from build123d import *

# Parameters (mm, degrees)
SKETCH1_W                       = 16
SKETCH1_H                       = 8
BOSS_EXTRUDE1_DEPTH             = 3
SHELL3_T                        = -1
SKETCH2_R                       = 1.5
SKETCH2_R_2                     = 0.8
BOSS_EXTRUDE2_DEPTH             = 2
BOSS_EXTRUDE3_DEPTH             = 11
CUT_EXTRUDE2_DEPTH              = 10
SKETCH5_R                       = 1.2
BOSS_EXTRUDE4_DEPTH             = 5
BOSS_EXTRUDE4_DIRECTION_2_REACH = 32.577


with BuildPart() as part:
    # Sketch1 → Boss-Extrude1 (new body)
    with BuildSketch(Plane.XY):
        with Locations((-13.569515058, 18.04477027)):
            Rectangle(SKETCH1_W, SKETCH1_H)
    extrude(amount=BOSS_EXTRUDE1_DEPTH)

    # Shell3
    shell3_openings = [part.faces().sort_by_distance(p)[0] for p in [
        (-13.569515058, 18.04477027, 0),
    ]]
    offset(amount=SHELL3_T, openings=shell3_openings, kind=Kind.INTERSECTION)

    # Sketch2 → Boss-Extrude2 (add)
    with BuildSketch(Plane(origin=(0, 0, 2), x_dir=(-1, 0, 0), z_dir=(0, 0, -1))):
        with Locations((13.569515058, 18.04477027)):
            Circle(SKETCH2_R)
        with Locations((13.569515058, 18.04477027)):
            Circle(SKETCH2_R_2, mode=Mode.SUBTRACT)
    extrude(amount=BOSS_EXTRUDE2_DEPTH)

    # Sketch3 → Boss-Extrude3 (add)
    with BuildSketch(Plane.XY.offset(3)):
        with BuildLine():
            Line((-17.569515058, 22.04477027), (-17.569515058, 20.54477027))
            Line((-17.569515058, 20.54477027), (-15.569515058, 20.54477027))
            ThreePointArc((-15.569515058, 20.54477027), (-13.569515058, 19.54477027), (-11.569515058, 20.54477027))
            Line((-11.569515058, 20.54477027), (-9.569515058, 20.54477027))
            Line((-9.569515058, 20.54477027), (-9.569515058, 22.04477027))
            Line((-9.569515058, 22.04477027), (-17.569515058, 22.04477027))
        make_face()
    extrude(amount=BOSS_EXTRUDE3_DEPTH)

    # Sketch4 → Cut-Extrude2 (cut)
    with BuildSketch(Plane.ZY.offset(17.569515058)):
        Polygon((14, 21.29477027), (14, 19.54477027), (10, 19.54477027), align=None)
    extrude(amount=-CUT_EXTRUDE2_DEPTH, mode=Mode.SUBTRACT)

    # Sketch5 → Boss-Extrude4 (add)
    with BuildSketch(Plane(origin=(0, 12.732659637, -5.570538591), x_dir=(-1, 0, 0), z_dir=(0, -0.9161573349021893, 0.4008188340197074))):
        with Locations(Location((13.569515058, -20.425962901, 0), (0, 0, 90))):
            Circle(SKETCH5_R)
    extrude(amount=BOSS_EXTRUDE4_DEPTH)

    # Sketch5 → Boss-Extrude4 direction 2 (add, up to next)
    with BuildSketch(Plane(origin=(0, 12.732659637, -5.570538591), x_dir=(-1, 0, 0), z_dir=(0, -0.9161573349021893, 0.4008188340197074)), mode=Mode.PRIVATE) as boss_extrude4_direction_2_sk1:
        with Locations(Location((13.569515058, -20.425962901, 0), (0, 0, 90))):
            Circle(SKETCH5_R)
    boss_extrude4_direction_2_tool1 = extrude(boss_extrude4_direction_2_sk1.sketch, amount=-BOSS_EXTRUDE4_DIRECTION_2_REACH, mode=Mode.PRIVATE) - part.part
    add(boss_extrude4_direction_2_tool1.solids().sort_by_distance((-13.569515, 20.91977, 13.142857))[0])


solid = part.part
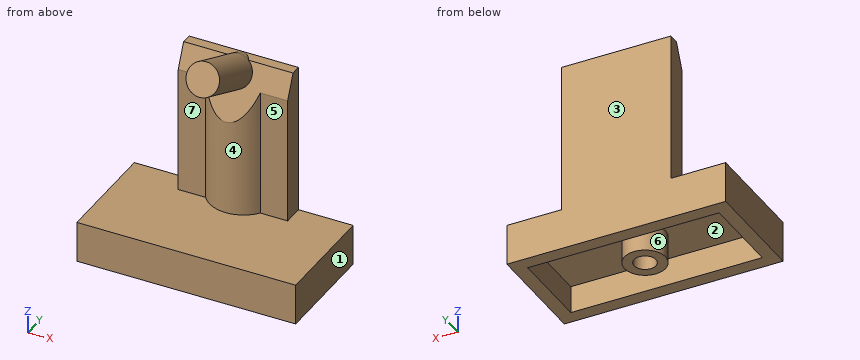
Read the model definition and answer for the solid it produces. Units are mm, in the model's axes. Face numbers are marked on the shaded views. A direction names the side the tool comes from. Coordinates: 2 decimals unless noted, no trailing zeros. Loops run counter-clockwise (first coordinate to the right, second up) from the corner with the lowest first, then second, coordinate; pieces in that order, holes last. Notation, with made-up numbers: (49.25, -32) - (98.25, -32) arc R30 ccw to (98.25, -8) - close; hole circle Ø10 at (-30, 87.5). An arc over 180 degrees is marked (long way). Answer in a Markdown table with one row per item.
Q1. Find section B-B on z = 6.25. Write down the section's boundary in (x, y).
Here are the results:
| item | result |
|---|---|
| outline | (-17.57, 20.54) - (-15.57, 20.54) arc R2.5 ccw to (-11.57, 20.54) - (-9.57, 20.54) - (-9.57, 22.04) - (-17.57, 22.04) - close |
Q2. Find section C-C on x = -19.5. Write down the section's boundary in (y, z), plus the area to 3 significant figures.
Here are the results:
| item | result |
|---|---|
| outline | (14.04, 0) - (15.04, 0) - (15.04, 2) - (21.04, 2) - (21.04, 0) - (22.04, 0) - (22.04, 3) - (14.04, 3) - close |
| area | 12.0 mm^2 |
Q3. The mould has two halves that part along Y. Classify the marked faces 1, 2 and 3: pulls with the +Y half, pulls with the -Y half, needs draft (parallel to the pull), parting line crosses it, or undercut.
Here are the results:
| item | result |
|---|---|
| face 1 | needs draft |
| face 2 | undercut |
| face 3 | pulls with the +Y half |
Q4. For the marked faces 4, 5, 6 and 7, determine the directions among +Z, -Z, +X, -X, +Y, -Y from which every point of the face is accessible in a straight line to the end or side of a thin tool.
Here are the results:
| item | result |
|---|---|
| face 4 | -Y |
| face 5 | +Z, +X, -Y |
| face 6 | -Z |
| face 7 | +Z, -X, -Y |
Q5. Find section D-D on y = 14.5. Write down the section's boundary in (x, z), plus the area to 3 significant figures.
Here are the results:
| item | result |
|---|---|
| outline | (-21.57, 0) - (-5.57, 0) - (-5.57, 3) - (-21.57, 3) - close |
| area | 48.0 mm^2 |
Q6. Find section A-A on x = -16.25. Write down the section's boundary in (y, z).
Here are the results:
| item | result |
|---|---|
| outline | (14.04, 0) - (15.04, 0) - (15.04, 2) - (21.04, 2) - (21.04, 0) - (22.04, 0) - (22.04, 14) - (21.29, 14) - (20.54, 12.29) - (20.54, 3) - (14.04, 3) - close |
Q7. Straight lines are drawn through the part: line 1 along Z through (x, y) = (-6.25, 18.25); line 2 along Z through (x, y) = (-15.25, 16.25); line 3 along Y through (x, z) = (-11.5, 6). For each, find the intervals that lie inside material, in ascending order. Write a range as [from, to].
Here are the results:
| item | result |
|---|---|
| line 1 | z = [0, 3] |
| line 2 | z = [2, 3] |
| line 3 | y = [20.54, 22.04] |
Q8. Given P1, Ø3, axis at x = -17, z = 10.5, coming from the -Y side; P2, Ø1.5, axis at x = -11, y = 18.5, coming from the +Z side; P3, Ø2.5, axis at x = -13, y = 19.5, coming from the +Z side; P4, Ø0.8, axis at x = -14, y = 18.5, coming from the -Z side, each flat-ended and moving along its own axis, determine where each tip first touches the part or whether it passes through.
Here are the results:
| item | result |
|---|---|
| P1 | stops at y = 20.46 |
| P2 | stops at z = 3 |
| P3 | stops at z = 15.58 |
| P4 | stops at z = 0 |
